Study the drawing (mm; zero at the part's minimum x, y, z) and answer. A direction names the side the tool comes from. Round coordinates to 2 decimals unless told otherwise and drop trailing zeros. Order: outer loops, then holes, each group sorted by start corner. A loop starts at its lowest first (then second) coordinate and runs counter-clockwise, first axis right, second up. Notation, with made-up numbers: (22.5, -2) -> (59.5, -2) arc R12 ccw to (59.5, 15) -> close; hole circle Ø4 at (22, 19). An arc over 180 degrees is marked (long way). Use one line per item in the form item = value.
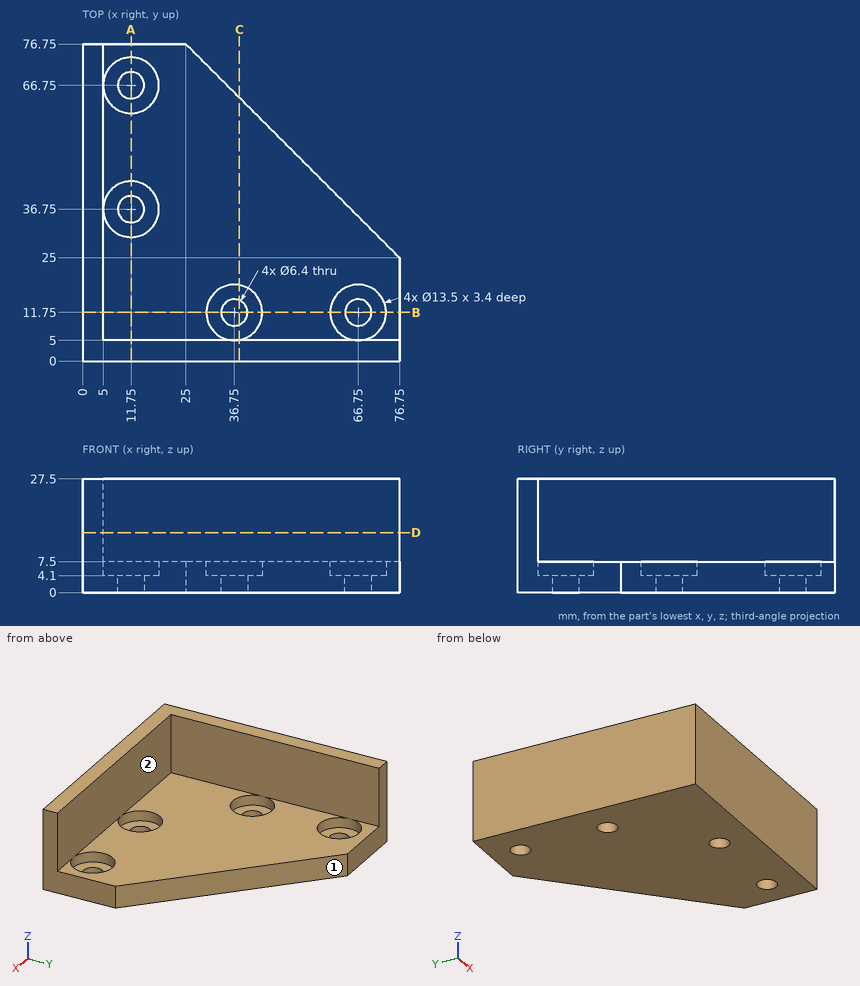
Item 1: The part is cut by section A-A, the plane x = 11.75. Give the vertices of the cut face in (y, z), and give its area (3 significant figures).
Findings:
outline = (0, 0) -> (33.55, 0) -> (33.55, 4.1) -> (30, 4.1) -> (30, 7.5) -> (5, 7.5) -> (5, 27.5) -> (0, 27.5) -> close; (39.95, 0) -> (63.55, 0) -> (63.55, 4.1) -> (60, 4.1) -> (60, 7.5) -> (43.5, 7.5) -> (43.5, 4.1) -> (39.95, 4.1) -> close; (69.95, 0) -> (76.75, 0) -> (76.75, 7.5) -> (73.5, 7.5) -> (73.5, 4.1) -> (69.95, 4.1) -> close
area = 531 mm^2
Item 2: The part is cut by section D-D, the plane z = 14.5. Give the vertices of the cut face in (x, y).
Findings:
outline = (0, 0) -> (76.75, 0) -> (76.75, 5) -> (5, 5) -> (5, 76.75) -> (0, 76.75) -> close
Item 3: The part is cut by section C-C, the plane x = 38. Give the vertices of the cut face in (y, z), and give its area (3 significant figures).
Findings:
outline = (0, 0) -> (8.8, 0) -> (8.8, 4.1) -> (5.12, 4.1) -> (5.12, 7.5) -> (5, 7.5) -> (5, 27.5) -> (0, 27.5) -> close; (14.7, 0) -> (63.75, 0) -> (63.75, 7.5) -> (18.38, 7.5) -> (18.38, 4.1) -> (14.7, 4.1) -> close
area = 509 mm^2
Item 4: Consider line 1 along Y through (x, z) = (11.75, 1.2); line 2 along X through (y, z) = (11.75, 6.75); line 3 along X through (y, z) = (31.5, 21.5). Determine where each line is inside the solid, lowest interval first.
Findings:
line_1 = 0 to 33.55, 39.95 to 63.55, 69.95 to 76.75
line_2 = 0 to 30, 43.5 to 60, 73.5 to 76.75
line_3 = 0 to 5
Item 5: Flat-ended cylindrical pins translate along their axes: P1, Ø16, axis at x = 27, z = 16, coming from the +Y side; P2, Ø1.5, axis at y = 31.5, z = 5, coming from the +X side; P3, Ø4, axis at x = 35.5, y = 13, coming from the +Z side; P4, Ø4, axis at x = 11.75, y = 66.75, coming from the -Z side. Find the tip coordinate at first contact, or state that the pin passes through.
Findings:
P1 = 5
P2 = 71
P3 = 4.1
P4 = through
Item 6: For the marked faces 1 and 2, determine the directions among +Z, -Z, +X, -X, +Y, -Y from which every point of the face is accessible in a straight line to the end or side of a thin tool.
Findings:
face_1 = +Z, -Z, +X, +Y
face_2 = +Z, +X, +Y
